Study the drawing (mm; zero at the part's minimum x, y, z) and answer. Round coordinates to 2 decimals unless told otherwise and drop trailing zeros. Write each loop counter-clockwise with the first axis right and the second up, starting at its lowest first coordinate (ties: lowest second). Pieces come first, ordered by that corner, then holes. Notation, with made-up numbers: (22, 79) - (75, 79) arc R15 ccw to (75, 107) - close; hole circle Ø4 at (52, 30). An arc over 180 degrees is marked (long way). Use one line per item in the form item = value. Start each with the question number.
1) Consider line 1 along Y through (x, z) = (1, 11) (3 decimals); line 2 along Y through (x, z) = (2.5, 9.5); line 3 along Z through (x, y) = (2.75, 35.5) (3 decimals). Determine where each line is inside the solid, lowest interval first. Write a range as from..to.
2) This flat-tipped pin is pushed along its axis until it touches: pin 1 (1.5 mm diameter, centred on x = 6, z = 5, fed in from -Y). Where does it stop, or does it pass through?
3) The part is cut by section A-A, the plane y = 35.5. Give the vertices of the cut face in (x, z) (3 decimals).
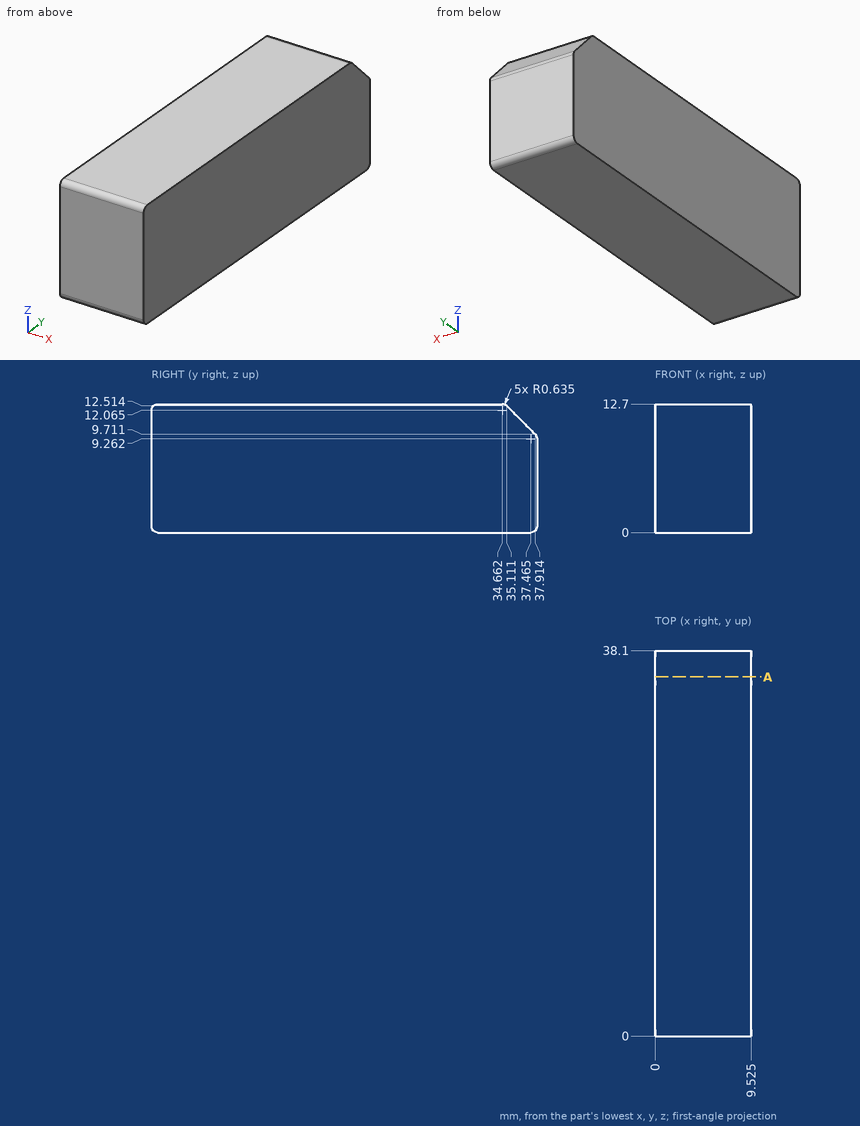
Geometry results:
q1.line_1 = 0..36.625
q1.line_2 = 0..38.05
q1.line_3 = 0..12.125
q2.pin_1 = 0
q3.outline = (0, 0) - (9.525, 0) - (9.525, 12.125) - (0, 12.125) - close
